The listing builds one solid part. Answer for the finished solid, in the listing's coordinates (mm). Round coordinates to 2 decimals unless told otherwise and drop trailing zeros. Write each loop counter-clockwise with the first axis right and the second up, starting at its lowest first coordinate (ties: lowest second). Pieces come first, ordered by that corner, then holes.
Item 1: Find section A-A on z = 172.5. Give the vertices of the cut face in (x, y), then the cut area to 3 significant figures.
Item 2: Each of these flat-tipped pins is pushed along its axis until it touches: pin 1 (5 mm diameter, centred on x = 140, z = 403, fed in from -Y); pin 2 (10 mm diameter, centred on x = 35.5, y = -6.5, fed in from -Z); pin 3 (1 mm diameter, centred on x = 74.5, y = -3, fed in from +Z); pin 4 (2 mm diameter, centred on x = 30.5, y = 7.5, fed in from +Z). Where does it stop, or does it pass through?
Item 3: Find the intervals of material crossed by probe 1 along Y at (x, z) = (130, 493); probe 2 along X at (y, z) = (-5.5, 916); probe 3 along Z at (x, y) = (111, -1.75), in increasing order.
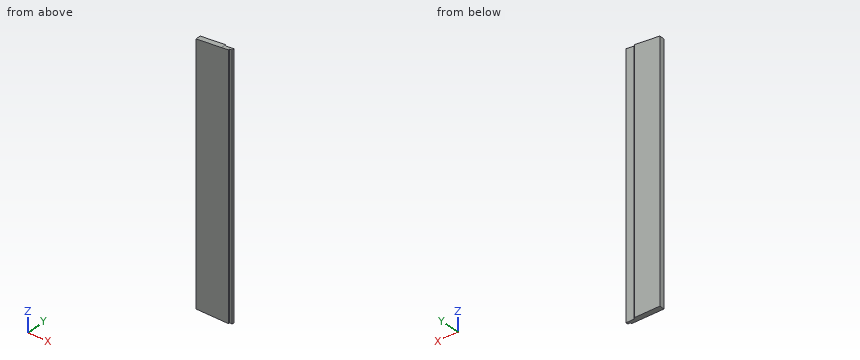
```python
from build123d import *

# Parameters (mm, degrees)
F1_DEPTH = 1100
F3_DEPTH = 1100.001
F5_DEPTH = 19.001


with BuildPart() as f1:
    # F0 (on Top) → F1 (new body)
    with BuildSketch(Plane.XY):
        Polygon((0, -4), (0, -9.5), (136, -9.5), (136, -4), (146, -4), (146, 4), (116, 4), (110.5, 9.5), (0, 9.5), (0, 4), (12, 4), (12, -4), align=None)
    extrude(amount=F1_DEPTH)

    # F2 (on face) → F3 (cut, through all)
    with BuildSketch(Plane(origin=(0, 0, 0), x_dir=(1, 0, 0), z_dir=(0, 0, -1))):
        Polygon((0, -9.5), (16, -9.5), (16, 9.5), (0, 9.5), (0, 4), (12, 4), (12, -4), (0, -4), align=None)
    extrude(amount=-F3_DEPTH, mode=Mode.SUBTRACT)

    # F4 (on face) → F5 (cut, through all)
    with BuildSketch(Plane(origin=(0, 9.5, 0), x_dir=(-1, 0, 0), z_dir=(0, 1, 0))):
        Polygon((-110.5, 1100), (-1424.1546681334, 1100), (-110.5, 961.9293307027), align=None)
        Polygon((-16, 1100), (-16, 951.99698047), (3, 950), (3, 1100), align=None)
        Polygon((-110.5, 1100), (-110.5, 961.9293307027), (-16, 951.99698047), (-16, 1100), align=None)
    extrude(amount=-F5_DEPTH, mode=Mode.SUBTRACT)


solid = f1.part
```
Check values:
1. outline: (16, -9.5) - (136, -9.5) - (136, -4) - (146, -4) - (146, 4) - (116, 4) - (110.5, 9.5) - (16, 9.5) - close
1. area: 2,230 mm2
2. pin 1: stops at y = -4
2. pin 2: stops at z = 0
2. pin 3: stops at z = 958.2
2. pin 4: stops at z = 953.63
3. probe 1: y = -9.5 to 4
3. probe 2: x = 16 to 136
3. probe 3: z = 0 to 961.98
